from build123d import *

# Parameters (mm, degrees)
BOSS_EXTRUDE1_DEPTH = 3
BOSS_EXTRUDE2_DEPTH = 3


with BuildPart() as part:
    # Sketch1 → Boss-Extrude1 (new body)
    with BuildSketch(Plane.XY):
        Polygon((-381, 211.461110197), (0, 0), (0, 38.1), (-381, 249.561110197), align=None)
    extrude(amount=BOSS_EXTRUDE1_DEPTH)

    # Sketch3 → Boss-Extrude2 (add)
    with BuildSketch(Plane.XY.offset(3)):
        Polygon((0, 0), (-25.4, 0), (-25.4, 14.097407346), align=None)
    extrude(amount=-BOSS_EXTRUDE2_DEPTH)


solid = part.part
Design review of the part built by this model. Coordinates are the model's own, in mm. Round coordinates to 2 decimals unless told otherwise and drop trailing zeros. Loops run counter-clockwise (first coordinate to the right, second up) from the corner with the lowest first, then second, coordinate; pieces in that order, holes last. Notation, with made-up numbers: (68, -0.5) - (77, -0.5) arc R13 ccw to (77, 19.5) - close; hole circle Ø7 at (65, 64). An arc over 180 degrees is marked (long way). One line per item, written item: value. Start each with the question number.
1) Consider section C-C on y = 227.5. Give the boundary of the cut face in (x, z).
2) To check wall thickness, follow L1, parallel to Y at x = -210, z = 0.75; L2, parallel to X at y = 89, z = 1.85; L3, parallel to Y at x = -352.5, z = 0.3. State the ranges of each line that lie inside material, in increasing order. Write a range as from..to.
3) Consider section B-B on x = -308. Give the boundary of the cut face in (y, z).
4) Consider section A-A on z = 0.95. Give the boundary of the cut face in (x, y), then the cut area to 3 significant figures.
5) Insertion check: pin 1 Ø1.5 at (y, z) = (9.5, 2) entering from -X. The pin has a flat end and moves straight along its axis. Give the tip position at first contact, or say it passes through.
Reported:
1. outline: (-381, 0) - (-341.25, 0) - (-341.25, 3) - (-381, 3) - close
2. L1: y = 116.55..154.65
2. L2: x = -160.36..-91.71
2. L3: y = 195.64..233.74
3. outline: (170.94, 0) - (209.04, 0) - (209.04, 3) - (170.94, 3) - close
4. outline: (-381, 211.46) - (-25.4, 14.1) - (-25.4, 0) - (0, 0) - (0, 38.1) - (-381, 249.56) - close
4. area: 14,700 mm^2
5. pin 1: stops at x = -25.4
